from build123d import *

# Parameters (mm, degrees)
CROQUIS1_W              = 56.8
CROQUIS1_H              = 20.82
SALIENTE_EXTRUIR1_DEPTH = 184
CROQUIS5_W              = 52.8
CROQUIS5_H              = 16.82
CORTAR_EXTRUIR5_DEPTH   = 184
CROQUIS6_R              = 1.5
CORTAR_EXTRUIR6_DEPTH   = 26


with BuildPart() as part:
    # Croquis1 → Saliente-Extruir1 (new body)
    with BuildSketch(Plane.XY):
        with Locations((8.738488477, -207.47377213)):
            Rectangle(CROQUIS1_W, CROQUIS1_H)
    extrude(amount=SALIENTE_EXTRUIR1_DEPTH)

    # Croquis5 → Cortar-Extruir5 (cut)
    with BuildSketch(Plane(origin=(0, 0, 0), x_dir=(-1, 0, 0), z_dir=(0, 0, -1))):
        with Locations((-8.738488477, -207.47377213)):
            Rectangle(CROQUIS5_W, CROQUIS5_H)
    extrude(amount=-CORTAR_EXTRUIR5_DEPTH, mode=Mode.SUBTRACT)

    # Croquis6 → Cortar-Extruir6 (cut)
    with BuildSketch(Plane(origin=(0, -197.06377213, 0), x_dir=(1, 0, 0), z_dir=(0, 1, 0))):
        with Locations((-3.261511523, -18)):
            Circle(CROQUIS6_R)
        with Locations((20.738488477, -18)):
            Circle(CROQUIS6_R)
        with Locations((-3.261511523, -166)):
            Circle(CROQUIS6_R)
        with Locations((20.738488477, -166)):
            Circle(CROQUIS6_R)
    extrude(amount=-CORTAR_EXTRUIR6_DEPTH, mode=Mode.SUBTRACT)


solid = part.part
The model under review builds one solid part; all positions refer to its coordinate system, in mm. A direction names the side the tool comes from. Give positions to 0.01 mm unless a question says otherwise; leave off trailing zeros. Loops run counter-clockwise (first coordinate to the right, second up) from the corner with the lowest first, then second, coordinate; pieces in that order, holes last. Notation, with made-up numbers: (10.25, -17) -> (35.25, -17) arc R31 ccw to (35.25, 12) -> close; hole circle Ø8 at (-10.5, 77). An arc over 180 degrees is marked (long way). Answer as a JSON object with one key per item and string values. Group by question number.
Q1. Tool access review of faces 1 (the flat face through (-17.662, -208, 91)), 2 (the flat face through (8.6, -198.9, 184)): name each direction out of +Z, -Z, +X, -X, +Y, -Y from which nothing blocks a thin tool from reaching the whole face with its end or side.
Q2. Take a section at B-B (z = 150). Write out the cut boundary in (x, y).
Q3. Take a section at C-C (x = 24). Write out the cut boundary in (y, z), plus the area to 3 significant figures.
Q4. Take a section at A-A (y = -208.25). Write out the cut boundary in (x, z), plus the area to 3 significant figures.
Q5. Wall thickness on line 1 along X through (y, z) = (-197.9, 18); line 2 along Y through (x, z) = (12.5, 168); line 3 along X through (y, z) = (-201.5, 158): over which ranges is each line inside the solid? List them lowest first.
Q6. Draft analysis for pull direction X (two halves, no side actions). For faces 3 (the cylindrical face through (20.543, -216.87, 164.513)), 4 (the flat face through (8, -197.064, 91)), 5 (the flat face through (-19.662, -208, 91)), state which applies: pulls with the +X half, pulls with the -X half, needs draft (parallel to the pull), parting line crosses it, or undercut.
Answer below:
{
 "1": {"face 1": "+Z, -Z", "face 2": "+Z, +X, -X, +Y, -Y"},
 "2": {"outline": "(-19.66, -217.88) -> (37.14, -217.88) -> (37.14, -197.06) -> (-19.66, -197.06) -> close; hole (-17.66, -215.88) -> (35.14, -215.88) -> (35.14, -199.06) -> (-17.66, -199.06) -> close"},
 "3": {"outline": "(-217.88, 0) -> (-215.88, 0) -> (-215.88, 184) -> (-217.88, 184) -> close; (-199.06, 0) -> (-197.06, 0) -> (-197.06, 184) -> (-199.06, 184) -> close", "area": "736 mm2"},
 "4": {"outline": "(-19.66, 0) -> (-17.66, 0) -> (-17.66, 184) -> (-19.66, 184) -> close; (35.14, 0) -> (37.14, 0) -> (37.14, 184) -> (35.14, 184) -> close", "area": "736 mm2"},
 "5": {"line 1": "x = -19.66 to -4.76, -1.76 to 19.24, 22.24 to 37.14", "line 2": "y = -217.88 to -215.88, -199.06 to -197.06", "line 3": "x = -19.66 to -17.66, 35.14 to 37.14"},
 "6": {"face 3": "undercut", "face 4": "needs draft", "face 5": "pulls with the -X half"}
}
